from build123d import *

# Parameters (mm, degrees)
SKETCH7_R             = 25.69
SKETCH7_W             = 8.6
SKETCH7_H             = 8.6
LENS_SPACER_DEPTH     = 7.08
SKETCH5_W             = 8.2
SKETCH5_H             = 24
SKETCH5_R             = 1.125
ATTACHMENT_LEGS_DEPTH = 1.5
LENS_START            = -7.08
SKETCH8_R             = 26.19
SKETCH8_R_2           = 25.69
LENS_POSITIONER_DEPTH = 8.09
SKETCH11_W            = 4
SKETCH11_H            = 3
NODE_HOLE_DEPTH       = 0.7


with BuildPart() as part:
    # Sketch7 → Lens Spacer (new body)
    with BuildSketch(Plane.XZ):
        with Locations(Location((0, 0, 0), (0, 0, 270))):
            Circle(SKETCH7_R)
        Rectangle(SKETCH7_W, SKETCH7_H, mode=Mode.SUBTRACT)
    extrude(amount=LENS_SPACER_DEPTH)

    # Sketch5 → Attachment Legs (add)
    # profile 1 of 2: a face of its own
    with BuildSketch(Plane(origin=(0, -7.08, 0), x_dir=(-1, 0, 0), z_dir=(0, -1, 0))):
        with Locations((-8.4, 2.1)):
            Rectangle(SKETCH5_W, SKETCH5_H)
        with Locations(Location((-10.75, 12.5, 0), (0, 0, 90))):
            Circle(SKETCH5_R, mode=Mode.SUBTRACT)
        with Locations(Location((-10.75, -0.3, 0), (0, 0, 90))):
            Circle(SKETCH5_R, mode=Mode.SUBTRACT)
    # profile 2 of 2: a face of its own
    with BuildSketch(Plane(origin=(0, -7.08, 0), x_dir=(-1, 0, 0), z_dir=(0, -1, 0))):
        with Locations((8.4, 2.1)):
            Rectangle(SKETCH5_W, SKETCH5_H)
        with Locations(Location((10.25, -0.3, 0), (0, 0, 270))):
            Circle(SKETCH5_R, mode=Mode.SUBTRACT)
        with Locations(Location((10.25, 12.5, 0), (0, 0, 270))):
            Circle(SKETCH5_R, mode=Mode.SUBTRACT)
    extrude(amount=ATTACHMENT_LEGS_DEPTH)

    # Sketch8 → Lens Positioner (add)
    with BuildSketch(Plane(origin=(0, 0, 0), x_dir=(1, 0, 0), z_dir=(0, 1, 0)).offset(LENS_START)):
        with Locations(Location((0, 0, 0), (0, 0, 270))):
            Circle(SKETCH8_R)
        with Locations(Location((0, 0, 0), (0, 0, 270))):
            Circle(SKETCH8_R_2, mode=Mode.SUBTRACT)
    extrude(amount=LENS_POSITIONER_DEPTH)

    # Sketch11 → Node Hole (cut)
    with BuildSketch(Plane.XZ.offset(8.58)):
        with Locations((7.9, -9.6)):
            Rectangle(SKETCH11_W, SKETCH11_H)
    extrude(amount=-NODE_HOLE_DEPTH, mode=Mode.SUBTRACT)

    # Sketch13 → Cut-Revolve1 (revolve, cut)
    with BuildSketch(Plane.XY, mode=Mode.PRIVATE) as cut_revolve1_sk:
        with BuildLine():
            Line((-7.7, -7.08), (-26.19, -7.08))
            Line((-26.19, -7.08), (-26.19, -1.79))
            ThreePointArc((-26.19, -1.79), (-18.616939408, -2.463282886), (-11.265314293, -4.401881538))
            ThreePointArc((-11.265314293, -4.401881538), (-9.27901976, -5.469843244), (-7.7, -7.08))
        make_face()
    revolve(cut_revolve1_sk.sketch.rotate(Axis((0, -81.156506397, 0), (0, 1, 0)), 270), axis=Axis((0, -81.156506397, 0), (0, 1, 0)), mode=Mode.SUBTRACT)


solid = part.part
For this review, take the finished solid that the model builds, in its own axes (mm). A direction names the side the tool comes from. Round coordinates to 2 decimals unless told otherwise and drop trailing zeros. Write item = value, one per line. Start each with the question number.
1) Insertion check: pin 1 (1.5 mm diameter, centred on x = -20, z = -11.5, fed in from +Y); pin 2 (1.6 mm diameter, centred on x = -9, y = -7.5, fed in from -Z); pin 3 (0.8 mm diameter, centred on y = -8, z = -9, fed in from +X). Each pin has a flat end and moves straight along its axis. Give the tip position at first contact, or say it passes through.
2) Take a section at A-A on z = -12.5. Count the separate pieces of the cut face and the enclosed holes in it, plus the area to 3 significant figures.
3) Tool access review of faces 1 (the face through (-25.08, 0.5, -5.57)), 2 (the face through (12.5, -8, -2)), 3 (the face through (0, -3, -4.3)), 4 (the face through (-9.15, -7.82, 0.06)), 5 (the face through (8, -8, 9.9)): name each direction out of +Z, -Z, +X, -X, +Y, -Y from which nothing blocks a thin tool from reaching the whole face with its end or side.
4) The part is to be moulded in two halves that separate along Z. For faces 6 (the face through (-9.252, -7.82, -11.981)), 7 (the face through (-8, -8, 9.9)), 8 (the face through (0, -7.08, -6)), say which applies: +Z half, -Z half, draft (parallel to the pull), parting line (faces both ways), or undercut.
5) To check wall thickness, follow line 1 (X direction, y = -7.85, z = -12.5) (3 decimals); line 2 (X direction, y = -8, z = -8.5); line 3 (Z direction, x = -10.25, y = -8.15) (3 decimals). State the ranges of each line that lie inside material, in increasing order. Write a range as from..to.
Verdict:
q1.pin_1 = 0
q1.pin_2 = -14.1
q1.pin_3 = 12.5
q2.separate_pieces = 5
q2.enclosed_holes = 0
q2.area = 149 mm2
q3.face_1 = +Y
q3.face_2 = +Z, -Z, +X, -Y
q3.face_3 = +Y, -Y
q3.face_4 = -Y
q3.face_5 = +Z, +X, -X, -Y
q4.face_6 = undercut
q4.face_7 = +Z half
q4.face_8 = draft
q5.line_1 = -12.5..-11.375, -9.125..-4.3, 4.3..9.625, 11.875..12.5
q5.line_2 = -12.5..-4.3, 4.3..5.9, 9.9..12.5
q5.line_3 = -14.1..-13.625, -11.375..-0.825, 1.425..9.9
